Can you work these out from the model? Positions are in its coordinate system, mm. A direction names the side the tool comes from. Round coordinates to 2 decimals unless told otherwise and drop trailing zeros. Loops run counter-clockwise (first coordinate to the right, second up) from the corner with the lowest first, then second, coordinate; pieces in that order, holes last. Notation, with made-up numbers: (46, 59) -> (80, 59) arc R5 cw to (80, 66) -> close; hole circle Ø1 at (-25.75, 82). An arc over 180 degrees is marked (long way). Use a Markdown table: item, result.
Autodesk Inventor part; units mm, degrees
ref_plane "Work Plane1" through (1.525, 0, 0) normal (0, 0, 1) x (1, 0, 0)
ref_plane "YZ Plane" through (0, 0, 0) normal (1, 0, 0) x (0, 1, 0)
ref_plane "XZ Plane" through (0, 0, 0) normal (0, 1, 0) x (-1, 0, 0)
sketch "Náčrt1" plane through (0, 0, 0) normal (0, 0, 1) x (1, 0, 0)
  line L0 (0, 4) -> (30, 4)
  line L1 (30, 4) -> (30, 0)
  line L2 (30, 0) -> (0, 0)
  line L3 (-6, 0) -> (36, 0)
  line L4 (0, -0.8) -> (0, 4.8)
  line L5 (0, 4) -> (0, 0)
  dimension "d2" = 8
  dimension "d59" = 30
revolve "Těleso" add sketch "Náčrt1" angle 360 about axis through (30, 0, 0) along (-1, 0, 0)
sketch "Náčrt2" plane through (0, 0, 0) normal (-1, 0, 0) x (0, 0, 1)
  line L0 (0, 6.9282) -> (6, 3.4641)
  line L1 (6, 3.4641) -> (6, -3.4641)
  line L2 (6, -3.4641) -> (0, -6.9282)
  line L3 (0, -6.9282) -> (-6, -3.4641)
  line L4 (-6, -3.4641) -> (-6, 3.4641)
  line L5 (-6, 3.4641) -> (0, 6.9282)
  line L6 (-8.4, 0) -> (8.4, 0)
  line L7 (0, 9.6995) -> (0, -9.6995)
  point P0 (0, 0)
  point P1 (0, 0)
  dimension "d11" = 12
extrude "Hlava" add sketch "Náčrt2" along normal blind 5
sketch "Náčrt4" plane through (0, 0, 0) normal (0, 0, 1) x (1, 0, 0)
  line L0 (-4.3072, 7.2) -> (-5, 6)
  line L1 (-1.1, 0) -> (-0.234, 0)
  line L2 (-5.9532, 0) -> (0.7192, 0)
  line L3 (-5, 7.2) -> (-4.3072, 7.2)
  line L4 (-5, 6) -> (-5, 7.2)
  line L5 (0, 8.64) -> (0, -1.44)
  dimension "d65" = 12
  dimension "d67" = 30
  dimension "d68" = 14.4
  dimension "d69" = 5
revolve "Zkosení1" cut sketch "Náčrt4" angle 360 about axis through (-1.1, 0, 0) along (1, 0, 0)
thread "Závit"
chamfer "Zkosení2" distance 0.7668 distance2 0.7669 1 edges at (30, -4, 0) measured on face at (30, -0.998, 0.8842)
fillet "Fillet2" radius 0.5 1 edges at (0, -4, 0)
ref_plane "Work Plane1" through (1.525, 0, 0) normal (0, 0, 1) x (1, 0, 0)
equation "\"d2\" = GD"
equation "\"d59\" = NLG"
equation "\"d11\" = SW"
equation "\"d3\" = KOH"
equation "\"d71\" = RR"
equation "\"d15\" = GEL"
equation "\"d6\" = -0.5 * SPD + 0.5 * GD"
equation "\"d65\" = SW"
equation "\"d67\" = ANG1"
equation "\"d68\" = 1.2 * SW"
equation "\"d69\" = KOH"
equation "\"NLG\" = 30"
equation "\"GD\" = NND"
equation "\"BDM\" = NND"
equation "\"KOH\" = 5"
equation "\"GEL\" = 14"
equation "\"SW\" = 12"
equation "\"SW0\" = 12"
equation "\"SPD\" = NND - 1.2269 * PTC"
equation "\"SD2\" = NND"
equation "\"SD\" = 0"
equation "\"ANG1\" = 30deg"
equation "\"GAL\" = 0.61345 * PTC"
equation "\"GUL\" = 0.61345 * PTC"
equation "\"RR\" = 0.5"
equation "\"RR1\" = 0.1"
equation "\"GD1\" = THREADDIA - 1.2269 * PTC"
equation "\"THREADDIA\" = 8"
equation "\"TOA\" = 30deg"
equation "\"FAWI\" = 60deg"
equation "\"PTC\" = 1.25"
equation "\"NND\" = 8"
equation "\"E0\" = 1.155 * SW"
properties part number "CSN 02 1201 - M8 x 30" material "Nerezová ocel"
1. Which directions (+Z, -Z, +X, -X, +Y, -Y) give clear straight access to the entire face, cutting with the end or side of a thin tool? Please do faces 4 (the flat face through (0, -5, 0)), 5 (the flat face through (-2, 0, 6)).
Answer sheet:
| item | result |
|---|---|
| face 4 | +X |
| face 5 | +Z, +X, -X, +Y, -Y |
2. I want a section at A-A (x = 4). Please give me the cut outline in (y, z), plus the area to 3 significant figures.
Answer sheet:
| item | result |
|---|---|
| outline | circle Ø8 at (0, 0) |
| area | 50.3 mm² |
3. If we mould it in two halves opening along Z, with no side actions, what happens to faces 1 (the conical face through (-4.87, -6.226, 0.015)), 2 (the conical face through (-4.87, -3.1, 5.4)), 3 (the flat face through (-5, 0, 0))? For each: +Z half, -Z half, draft (parallel to the pull), parting line (faces both ways), or undercut.
Answer sheet:
| item | result |
|---|---|
| face 1 | parting line |
| face 2 | +Z half |
| face 3 | draft |
4. I need wall thicknesses on line 1 (Z direction, x = 16.5, y = -2); line 2 (X direction, y = -4.75, z = 0.5); line 3 (Z direction, x = 12, y = 0.25). Which ranges of each line are inside material? Lowest first, please.
Answer sheet:
| item | result |
|---|---|
| line 1 | z = -3.46 to 3.46 |
| line 2 | x = -5 to 0 |
| line 3 | z = -3.99 to 3.99 |
5. Will these pins go through, and if not, where does the flat tip stop? pin 1 Ø1.5 at (x, y) = (12, -2.5) entering from -Z; pin 2 Ø1 at (x, z) = (2.5, -1.5) entering from +Y; pin 3 Ø3 at (x, z) = (15.5, 1) entering from +Y.
Answer sheet:
| item | result |
|---|---|
| pin 1 | stops at z = -3.6 |
| pin 2 | stops at y = 3.87 |
| pin 3 | stops at y = 4 |
